```python
from build123d import *

# Parameters (mm, degrees)
BOSS_EXTRUDE1_DEPTH     = 300
SKETCH3_R               = 15.5
CUT_EXTRUDE1_DEPTH      = 23
CUT_EXTRUDE1_DEPTH_BACK = 23
SKETCH4_R               = 35
CUT_EXTRUDE3_DEPTH      = 300
SKETCH5_W               = 541.558659161
SKETCH5_H               = 211.066516127
SKETCH5_W_2             = 529.372370701
SKETCH5_H_2             = 106.264435371
CUT_EXTRUDE4_DEPTH      = 201.0000001


with BuildPart() as part:
    # Sketch1 → Boss-Extrude1 (new body)
    with BuildSketch(Plane(origin=(0, 0, 0), x_dir=(1, 0, 0), z_dir=(0, 1, 0))):
        with BuildLine():
            Line((-200, 1e-09), (200, 1e-09))
            add(Edge.make_bspline(
                [(-200, 1e-09), (0, -400.000000001), (200, 1e-09)],
                knots=[0.056028396, 0.056028396, 0.056028396, 0.943971604, 0.943971604, 0.943971604], degree=2))
        make_face()
    extrude(amount=BOSS_EXTRUDE1_DEPTH)

    # Sketch3 → Cut-Extrude1 (cut, two sides)
    with BuildSketch(Plane(origin=(0, 150, 0), x_dir=(1, 0, 0), z_dir=(0, 1, 0))) as cut_extrude1_sk:
        with Locations((0, -142.999999999)):
            Circle(SKETCH3_R)
    extrude(amount=CUT_EXTRUDE1_DEPTH, mode=Mode.SUBTRACT)
    extrude(cut_extrude1_sk.sketch, amount=-CUT_EXTRUDE1_DEPTH_BACK, mode=Mode.SUBTRACT)

    # Sketch4 → Cut-Extrude3 (cut)
    with BuildSketch(Plane(origin=(0, 173, 0), x_dir=(1, 0, 0), z_dir=(0, 1, 0))):
        with Locations((0, -142.999999999)):
            Circle(SKETCH4_R)
    cut_extrude3 = extrude(amount=CUT_EXTRUDE3_DEPTH, mode=Mode.SUBTRACT)

    # Mirror1: Cut-Extrude3 across plane
    add(cut_extrude3.mirror(Plane.ZX.offset(150)), mode=Mode.SUBTRACT)

    # Sketch5 → Cut-Extrude4 (cut, through all)
    with BuildSketch(Plane(origin=(0, 0, 0), x_dir=(-1, 0, 0), z_dir=(0, 0, -1))):
        with Locations((21.44786769, 42.066741937)):
            Rectangle(SKETCH5_W, SKETCH5_H)
        with Locations((2.680983461, 251.532217686)):
            Rectangle(SKETCH5_W_2, SKETCH5_H_2)
    extrude(amount=-CUT_EXTRUDE4_DEPTH, mode=Mode.SUBTRACT)


solid = part.part
```
Verification items for the finished model (mm, model axes). A direction names the side the tool comes from. Round coordinates to 2 decimals unless told otherwise and drop trailing zeros.
1. Gauge pin test, flat ends, axial feed: P1, Ø4, axis at y = 168.5, z = 93, coming from the -X side; P2, Ø10, axis at x = 92.5, y = 184.5, coming from the +Z side; P3, Ø1.5, axis at y = 153, z = 145.5, coming from the +X side. Record the tip position at first contact, or that the pin passes through.
2. Draft check along X on faces 1 (the cylindrical face through (-7.587, 185.522, 177.168)), 2 (the flat face through (3, 147.6, 76)). Enter one of: +X half, -X half, draft (parallel to the pull), parting line (faces both ways), or undercut.
3. Scan lines: L1, parallel to Z at x = 0, y = 161; L2, parallel to Z at x = 0, y = 180; L3, parallel to X at y = 181, z = 143. Record each from-to range of solid material in increasing order.
4. Access from +Z, -Z, +X, -X, +Y, -Y to the whole of each face (thin tool, end or side, straight path). Record for faces 3 (the flat face through (3, 198.4, 76)), 4 (the flat face through (15, 173, 150)).
Answer:
1. P1: stops at x = -147.65
1. P2: stops at z = 161.72
1. P3: stops at x = 105.12
2. face 1: undercut
2. face 2: draft
3. L1: z = 0 to 127.5, 158.5 to 200
3. L2: z = 0 to 108, 178 to 200
3. L3: x = -106.77 to -35, 35 to 106.77
4. face 3: +Z, -Z, +X, -X, +Y
4. face 4: +Y
